Could you check a few things on this drawing? It's one solid part, dimensions in mm from its lowest x, y, z. Give positions to 0.01 mm unless a question says otherwise; leave off trailing zeros. Order: outer loops, then holes, each group sorted by start corner. A loop starts at its lowest first (then second) coordinate and runs counter-clockwise, first axis right, second up. Notation, with made-up numbers: (7, 60) - (19, 60) arc R21 cw to (19, 71) - close; hole circle Ø6 at (6, 68). An arc over 180 degrees is marked (long way). Return JSON: item names as keys, results as strings.
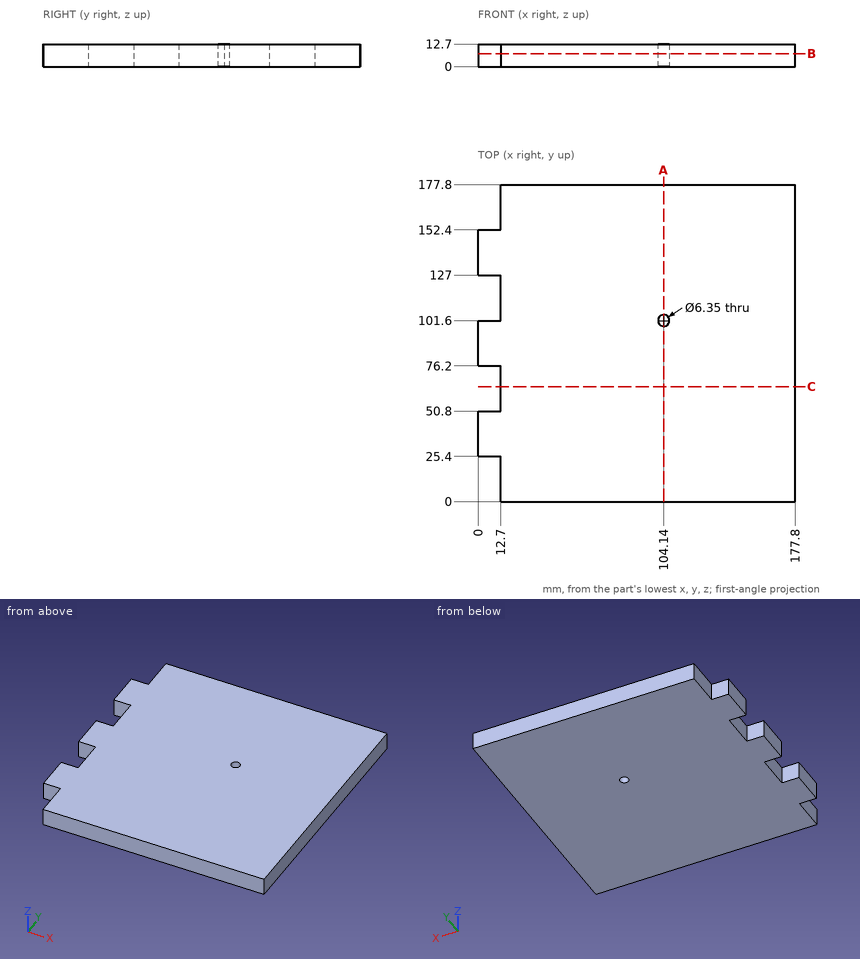
1. For pin 1 Ø6.5 at (y, z) = (68, 8) entering from -X; pin 2 Ø6.5 at (x, z) = (6.5, 6) entering from +Y, each with a flat end and sliding along its axis, tell me the tip position at first contact or that it passes through.
Checks:
{"pin 1": "x = 12.7", "pin 2": "y = 152.4"}
2. Suppose I cut it at A-A (x = 104.14). List the corners of the cut face in (y, z) for me (3 decimals).
Checks:
{"outline": "(0, 0) - (98.425, 0) - (98.425, 12.7) - (0, 12.7) - close; (104.775, 0) - (177.8, 0) - (177.8, 12.7) - (104.775, 12.7) - close"}
3. Suppose I cut it at B-B (z = 7.25). List the corners of the cut face in (x, y) for me (3 decimals).
Checks:
{"outline": "(0, 25.4) - (12.7, 25.4) - (12.7, 0) - (177.8, 0) - (177.8, 177.8) - (12.7, 177.8) - (12.7, 152.4) - (0, 152.4) - (0, 127) - (12.7, 127) - (12.7, 101.6) - (0, 101.6) - (0, 76.2) - (12.7, 76.2) - (12.7, 50.8) - (0, 50.8) - close; hole circle Ø6.35 at (104.14, 101.6)"}
4. If I drill on L1, parallel to Y at x = 104.14, z = 8.75 (3 decimals); L2, parallel to X at y = 103, z = 12; L3, parallel to X at y = 126, z = 3, over which ranges is the centre line in solid material (lowest first)? Write a range as [from, to].
Checks:
{"L1": "[0, 98.425], [104.775, 177.8]", "L2": "[12.7, 101.29], [106.99, 177.8]", "L3": "[12.7, 177.8]"}
5. Suppose I cut it at C-C (y = 64.5). List the corners of the cut face in (x, z) for me.
Checks:
{"outline": "(12.7, 0) - (177.8, 0) - (177.8, 12.7) - (12.7, 12.7) - close"}
